```python
from build123d import *

# Parameters (mm, degrees)
F0_R           = 1
F1_DEPTH       = 2
F3_D           = 2.5
F3_DEPTH       = 15.81
F3_CSINK_D     = 5
F3_CSINK_ANGLE = 90
F3_TIP         = 0.7510757738


# Not quite as in the source:
# - a feature names something its author has since deleted; it is built from what else it names


with BuildPart() as f1:
    # F0 (on Top) → F1 (new body)
    with BuildSketch(Plane.XY):
        with BuildLine():
            Line((-8.0353952667, -6.0930074749), (8.4878063746, -5.4451317825))
            ThreePointArc((8.4878063746, -5.4451317825), (9.3335768433, -4.9115848639), (9.2943968921, -3.912352693))
            Line((9.2943968921, -3.912352693), (0.4717192633, 10.0732218341))
            ThreePointArc((0.4717192633, 10.0732218341), (-0.4132311567, 10.5389070865), (-1.2590016254, 10.0053601679))
            Line((-1.2590016254, 10.0053601679), (-8.9595256379, -4.6280900516))
            ThreePointArc((-8.9595256379, -4.6280900516), (-8.9203456867, -5.6273222225), (-8.0353952667, -6.0930074749))
        make_face()
        with Locations((-0.2769940404, 7.0643619393)):
            Circle(F0_R, mode=Mode.SUBTRACT)
    extrude(amount=F1_DEPTH)

    # F3
    with Locations(Plane.XY.offset(2)):
        with Locations((0.0693653225, -1.7690696287)):
            CounterSinkHole(F3_D / 2, F3_CSINK_D / 2, depth=F3_DEPTH, counter_sink_angle=F3_CSINK_ANGLE)
            with Locations((0, 0, -(F3_DEPTH + F3_TIP / 2))):  # 118° drill point
                Cone(0, F3_D / 2, F3_TIP, mode=Mode.SUBTRACT)


solid = f1.part
```
The listing builds one solid part. Answer for the finished solid, in the listing's coordinates (mm). Coordinates: 2 decimals unless noted, no trailing zeros. Write each loop counter-clockwise with the first axis right and the second up, starting at its lowest first coordinate (ties: lowest second). Pieces come first, ordered by that corner, then holes. Notation, with made-up numbers: (89, 17.25) - (126, 17.25) arc R9 cw to (126, 27.25) - close; hole circle Ø1 at (-13.75, -20). An arc over 180 degrees is marked (long way). Return JSON: item names as keys, results as strings. Group by question number.
1. A cutting plane is placed at C-C, the plane x = 0.25. Give the number of separate pieces and of enclosed holes in the cut face, plus the area to 3 significant figures.
2. A cutting plane is placed at B-B, the plane z = 1.15. Determine the outline of the cut face in (x, y), plus the area to 3 significant figures.
3. Straight lines are drawn through the part: L1, parallel to Y at x = 0.5, z = 1.15; L2, parallel to Y at x = 0.25, z = 1.8; L3, parallel to X at y = -1.5, z = 0.55. For each, find the intervals that lie inside material, in ascending order.
4. A cutting plane is placed at D-D, the plane x = -4.25. Determine the outline of the cut face in (y, z).
5. A cutting plane is placed at A-A, the plane y = 7.5. Determine the outline of the cut face in (x, z).
6. Determine the mould class of faces 1 (the flat face through (4.945, 2.983, 0.986)), 2 (the cylindrical face through (-0.494, 6.088, 0.986)), 3 (the cylindrical face through (-0.4, 10.54, 0.99)) for opening direction X: released by +X, released by -X, zero draft, split by the parting line, or undercut.
7. Given pin 1 (1 mm diameter, centred on y = 2.5, z = 1.5, fed in from +X), flat-ended and moving along its own axis, determine where the tip first touches the part or whether it passes through.
Ans:
{
 "1": {"separate pieces": "3", "enclosed holes": "0", "area": "22.3 mm²"},
 "2": {"outline": "(-8.96, -4.63) arc R1 ccw to (-8.04, -6.09) - (8.49, -5.45) arc R1 ccw to (9.29, -3.91) - (0.47, 10.07) arc R1 ccw to (-1.26, 10.01) - close; hole circle Ø3.3 at (0.07, -1.77); hole circle Ø2 at (-0.28, 7.06)", "area": "159 mm²"},
 "3": {"L1": "-5.76 to -3.36, -0.18 to 6.43, 7.69 to 10.03", "L2": "-5.77 to -4.06, 0.52 to 6.21, 7.91 to 10.32", "L3": "-7.31 to -1.15, 1.29 to 7.77"},
 "4": {"outline": "(-5.94, 0) - (4.32, 0) - (4.32, 2) - (-5.94, 2) - close"},
 "5": {"outline": "(-2.58, 0) - (-1.18, 0) - (-1.18, 2) - (-2.58, 2) - close; (0.62, 0) - (2.1, 0) - (2.1, 2) - (0.62, 2) - close"},
 "6": {"face 1": "released by +X", "face 2": "undercut", "face 3": "split by the parting line"},
 "7": {"pin 1": "x = 5.56"}
}
